Design review of the part built by this model. Coordinates are the model's own, in mm. A direction names the side the tool comes from. Give positions to 0.01 mm unless a question says otherwise; leave off trailing zeros. Loops run counter-clockwise (first coordinate to the right, second up) from the corner with the lowest first, then second, coordinate; pieces in that order, holes last.
from build123d import *

# Parameters (mm, degrees)
SKETCH1_R               = 1
BOSS_EXTRUDE1_DEPTH     = 1.6
SKETCH2_R               = 8.931361996
BOSS_EXTRUDE2_DEPTH     = 8.4
SKETCH3_W               = 8
SKETCH3_H               = 1.9
CUT_EXTRUDE1_DEPTH      = 9.4
CUT_EXTRUDE1_DEPTH_BACK = 2.6


with BuildPart() as part:
    # Sketch1 → Boss-Extrude1 (new body)
    with BuildSketch(Plane(origin=(0, 0, 0), x_dir=(1, 0, 0), z_dir=(0, 1, 0))):
        with BuildLine():
            Line((10.779760555, 11.9), (-0.580107175, 11.9))
            ThreePointArc((-0.580107175, 11.9), (-2.930107175, 9.55), (-5.280107175, 11.9))
            Line((-5.280107175, 11.9), (-30.920239445, 11.9))
            Line((-30.920239445, 11.9), (-30.920239445, -11.9))
            Line((-30.920239445, -11.9), (-5.280107175, -11.9))
            ThreePointArc((-5.280107175, -11.9), (-2.930107175, -9.55), (-0.580107175, -11.9))
            Line((-0.580107175, -11.9), (10.779760555, -11.9))
            Line((10.779760555, -11.9), (10.779760555, 11.9))
        make_face()
        with Locations((-21.020239445, -10)):
            Circle(SKETCH1_R, mode=Mode.SUBTRACT)
        with Locations((-21.020239445, 10)):
            Circle(SKETCH1_R, mode=Mode.SUBTRACT)
    extrude(amount=BOSS_EXTRUDE1_DEPTH)

    # Sketch2 → Boss-Extrude2 (add)
    with BuildSketch(Plane(origin=(0, 1.6, 0), x_dir=(1, 0, 0), z_dir=(0, 1, 0))):
        Circle(SKETCH2_R)
    extrude(amount=BOSS_EXTRUDE2_DEPTH)

    # Sketch3 → Cut-Extrude1 (cut, two sides)
    with BuildSketch(Plane(origin=(0, 1.6, 0), x_dir=(1, 0, 0), z_dir=(0, 1, 0))) as cut_extrude1_sk:
        with Locations((-26.920239445, 10.95)):
            Rectangle(SKETCH3_W, SKETCH3_H)
        with Locations((-26.920239445, -10.95)):
            Rectangle(SKETCH3_W, SKETCH3_H)
    extrude(amount=CUT_EXTRUDE1_DEPTH, mode=Mode.SUBTRACT)
    extrude(cut_extrude1_sk.sketch, amount=-CUT_EXTRUDE1_DEPTH_BACK, mode=Mode.SUBTRACT)


solid = part.part
Q1. Take a section at A-A (y = 1). Give the boundary of the cut face in (x, z).
Results:
outline: (-30.92, -10) - (-22.92, -10) - (-22.92, -11.9) - (-5.28, -11.9) arc R2.35 cw to (-0.58, -11.9) - (10.78, -11.9) - (10.78, 11.9) - (-0.58, 11.9) arc R2.35 cw to (-5.28, 11.9) - (-22.92, 11.9) - (-22.92, 10) - (-30.92, 10) - close; hole circle Ø2 at (-21.02, -10); hole circle Ø2 at (-21.02, 10)
Q2. Draft analysis for pull direction X (two halves, no side actions). For faces 1 (the face through (10.78, 1, 0)), 2 (the face through (-21.757, 0.789, 9.324)), 3 (the face through (0, 10, 0)), state which applies: pulls with the +X half, pulls with the -X half, needs draft (parallel to the pull), parting line crosses it, or undercut.
Results:
face 1: pulls with the +X half
face 2: undercut
face 3: needs draft
Q3. Take a section at C-C (x = 0). Give the boundary of the cut face in (y, z), plus the area to 3 significant figures.
Results:
outline: (0, -11.9) - (1.6, -11.9) - (1.6, -8.93) - (10, -8.93) - (10, 8.93) - (1.6, 8.93) - (1.6, 11.9) - (0, 11.9) - close
area: 188 mm2
Q4. Take a section at B-B (z = 0). Give the boundary of the cut face in (x, y).
Results:
outline: (-30.92, 0) - (10.78, 0) - (10.78, 1.6) - (8.93, 1.6) - (8.93, 10) - (-8.93, 10) - (-8.93, 1.6) - (-30.92, 1.6) - close
Q5. Tool access review of faces 4 (the face through (-27, 1, -10)), 5 (the face through (4.121, 5.741, 7.924)), 6 (the face through (-27, 1, 10)): name each direction out of +Z, -Z, +X, -X, +Y, -Y from which nothing blocks a thin tool from reaching the whole face with its end or side.
Results:
face 4: -Z, -X, +Y, -Y
face 5: +Y
face 6: +Z, -X, +Y, -Y
Q6. Take a section at D-D (z = -10.5). Give the boundary of the cut face in (x, y), plus the area to 3 significant figures.
Results:
outline: (-22.92, 0) - (-21.89, 0) - (-21.89, 1.6) - (-22.92, 1.6) - close; (-20.15, 0) - (-4.82, 0) - (-4.82, 1.6) - (-20.15, 1.6) - close; (-1.04, 0) - (10.78, 0) - (10.78, 1.6) - (-1.04, 1.6) - close
area: 45.1 mm2
Q7. Insertion check: pin 1 (2 mm diameter, centred on y = 8, z = -2, fed in from -X); pin 2 (3 mm diameter, centred on x = -21.02, z = -10, fed in from +Y); pin 3 (6 mm diameter, centred on y = 6, z = 4.5, fed in from -X); pin 4 (1.2 mm diameter, centred on x = -21.02, z = 10, fed in from +Y). Each pin has a flat end and moves straight along its axis. Give the tip position at first contact, or say it passes through.
Results:
pin 1: stops at x = -8.88
pin 2: stops at y = 1.6
pin 3: stops at x = -8.8
pin 4: passes through
Q8. Wall thickness on line 1 (Y direction, x = -26.5, z = 8.25); line 2 (Z direction, x = -29, y = 0.5); line 3 (Z direction, x = 2, y = 5.75): over which ranges is each line inside the solid? List them lowest first.
Results:
line 1: y = 0 to 1.6
line 2: z = -10 to 10
line 3: z = -8.7 to 8.7
